Read the model definition and answer for the solid it produces. Units are mm, in the model's axes. Face numbers are marked on the shaded views. Coordinates: 2 decimals unless noted, no trailing zeros. Loops run counter-clockwise (first coordinate to the right, second up) from the corner with the lowest first, then second, coordinate; pieces in that order, holes last.
Q1. Straight lines are drawn through the part: line 1 (X direction, y = 0, z = 34); line 2 (X direction, y = 0, z = 34.5); line 3 (Z direction, x = 19, y = 1.75). For each, find the intervals that lie inside material, in ascending order.
Q2. The mould has two halves that part along Y. Classify the marked faces 1, 2 and 3: pulls with the +Y half, pulls with the -Y half, needs draft (parallel to the pull), parting line crosses it, or undercut.
Q3. Section B-B (y = 7) is taken. Give the vertices of the cut face in (x, z).
Q4. Section D-D (z = -21.5) is taken. Give the vertices of the cut face in (x, y).
Q5. Flat-ended cylindrical pins translate along their axes: P1, Ø10, axis at y = 6, z = 21, coming from the -X side; P2, Ø6, axis at y = -0.5, z = -26.5, coming from the +X side; P3, Ø10, axis at y = -9, z = 12, coming from the +X side. Find the tip coordinate at first contact, or state that the pin passes through.
Q6. Section C-C (y = 0) is taken. Give the vertices of the cut face in (x, z).
Q7. Section A-A (x = 34) is taken. Give the vertices of the cut face in (y, z).
from build123d import *

# Parameters (mm, degrees)
F1_DEPTH = 12.7
F2_R     = 4
F3_DEPTH = 25.4


with BuildPart() as f1:
    # F0 (on Front) → F1 (new body, symmetric)
    with BuildSketch(Plane.XZ):
        Polygon((-37.331276, -25.252699), (-37.331276, -37.952699), (-24.631276, -37.952699), (46.483805, 38.328189), (24.792205, 38.328189), align=None)
    extrude(amount=F1_DEPTH, both=True)

    # F2 (on face) → F3 (cut)
    with BuildSketch(Plane.XY.offset(38.328189)):
        with Locations((34.659129, 0)):
            Circle(F2_R)
    extrude(amount=-F3_DEPTH, mode=Mode.SUBTRACT)


solid = f1.part
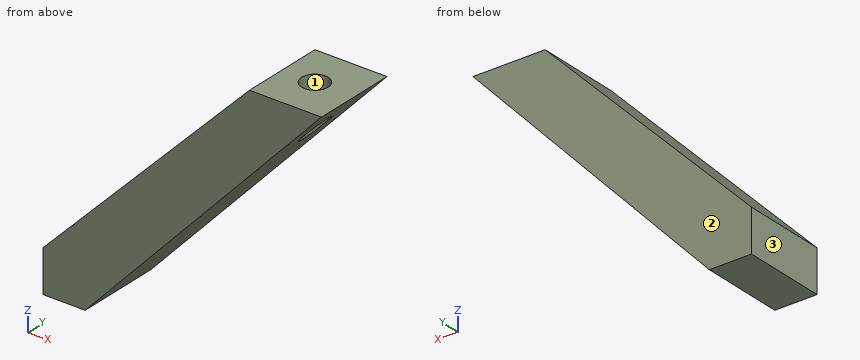
Numbers:
1. line 1: x = 20.56 to 30.66, 38.66 to 42.45
1. line 2: x = 21.05 to 30.66, 38.66 to 42.91
1. line 3: z = 8.85 to 32.4
2. face 1: undercut
2. face 2: pulls with the +Y half
2. face 3: needs draft
3. outline: (-37.33, -37.95) - (-24.63, -37.95) - (46.48, 38.33) - (24.79, 38.33) - (-37.33, -25.25) - close
4. outline: (-33.66, -12.7) - (-9.29, -12.7) - (-9.29, 12.7) - (-33.66, 12.7) - close
5. P1: stops at x = 2.98
5. P2: stops at x = -11.16
5. P3: stops at x = 26.6
6. outline: (-37.33, -37.95) - (-24.63, -37.95) - (30.66, 21.35) - (30.66, 38.33) - (24.79, 38.33) - (-37.33, -25.25) - close; (38.66, 29.94) - (46.48, 38.33) - (38.66, 38.33) - close
7. outline: (-12.7, 24.94) - (-3.95, 24.94) - (-3.95, 38.33) - (-12.7, 38.33) - close; (3.95, 24.94) - (12.7, 24.94) - (12.7, 38.33) - (3.95, 38.33) - close
